The listing builds one solid part. Answer for the finished solid, in the listing's coordinates (mm). Face numbers are marked on the shaded views. A direction names the side the tool comes from. Round coordinates to 2 decimals unless told otherwise and drop trailing zeros. Write each loop counter-clockwise with the first axis right and the second up, starting at its lowest first coordinate (ties: lowest second). Pieces come first, ordered by that corner, then holes.
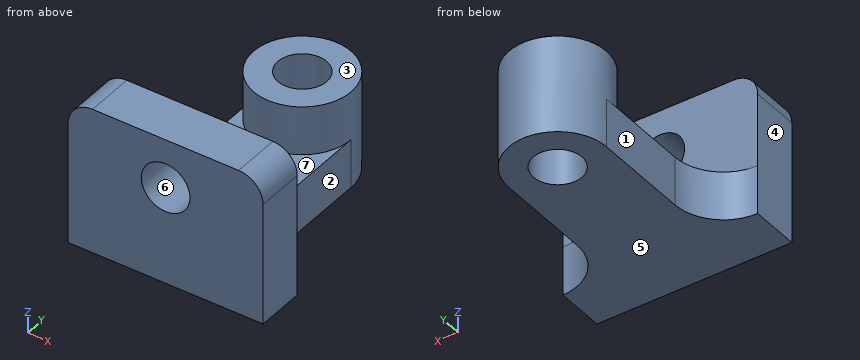
Autodesk Inventor part; units mm, degrees
ref_plane "YZ Plane" through (0, 0, 0) normal (1, 0, 0) x (0, 1, 0)
ref_plane "XZ Plane" through (0, 0, 0) normal (0, 1, 0) x (-1, 0, 0)
ref_plane "XY Plane" through (0, 0, 0) normal (0, 0, 1) x (1, 0, 0)
sketch "Sketch1" plane through (0, 0, 0) normal (0, 1, 0) x (-1, 0, 0)
  line L0 (28.0719, 23.0631) -> (-22.7281, 23.0631)
  line L1 (-22.7281, 23.0631) -> (-22.7281, -15.0369)
  line L2 (-22.7281, -15.0369) -> (28.0719, -15.0369)
  line L3 (28.0719, -15.0369) -> (28.0719, 23.0631)
  point P0 (0, 0)
  dimension "d0" = 50.8
  dimension "d1" = 38.1
extrude "Extrusion1" add sketch "Sketch1" along normal blind 12.7
sketch "Sketch2" plane through (0, 12.7, 0) normal (0, 1, 0) x (1, 0, 0)
  line L0 (22.7281, -23.0631) -> (22.7281, 15.0369)
  line L1 (22.7281, 15.0369) -> (10.0281, 15.0369)
  line L2 (10.0281, 15.0369) -> (10.0281, 2.3369)
  line L3 (10.0281, 2.3369) -> (22.7281, 2.3369)
  line L4 (22.7281, 2.3369) -> (22.7281, 15.0369)
  line L5 (22.7281, 15.0369) -> (-28.0719, 15.0369)
  line L6 (-28.0719, 15.0369) -> (-15.3719, 15.0369)
  line L7 (-15.3719, 15.0369) -> (-15.3719, 2.3369)
  line L8 (-15.3719, 2.3369) -> (-28.0719, 2.3369)
  line L9 (-28.0719, 2.3369) -> (-28.0719, 15.0369)
  line L10 (-15.3719, 15.0369) -> (10.0281, 15.0369)
  line L11 (10.0281, 15.0369) -> (10.0281, 2.3369)
  line L12 (10.0281, 2.3369) -> (-15.3719, 2.3369)
  line L13 (-15.3719, 2.3369) -> (-15.3719, 15.0369)
  point P0 (0, 0)
  dimension "d4" = 12.7
  dimension "d5" = 12.7
  dimension "d6" = 12.7
  dimension "d7" = 12.7
extrude "Extrusion2" add sketch "Sketch2" along normal blind 38.1 contours L12 L7 L5 L2
fillet "Fillet1" radius 12.7 1 edges at (10.0281, 12.7, -8.6869)
fillet "Fillet2" radius 12.7 1 edges at (-15.3719, 12.7, -8.6869)
sketch "Sketch3" plane through (22.7281, 0, -15.0369) normal (0, 0, -1) x (-1, 0, 0)
  line L0 (12.7, 25.4) -> (12.7, 50.8)
  line L1 (12.7, 50.8) -> (25.4, 50.8)
  line L2 (12.7, 50.8) -> (38.1, 50.8)
  circle A0 centre (25.4, 50.8) radius 12.7
  point P0 (22.7281, 0)
  dimension "d12" = 12.7
  dimension "d13" = 25.4
extrude "Extrusion3" add sketch "Sketch3" against normal blind 25.4
sketch "Sketch4" plane through (-2.6719, 50.8, 10.3631) normal (0, 0, 1) x (1, 0, 0)
  circle A0 centre (0, 0) radius 6.35
  point P0 (2.6719, -50.8)
  dimension "d16" = 12.7
extrude "Extrusion4" cut sketch "Sketch4" against normal blind 25.4
fillet "Fillet3" radius 6.35 1 edges at (22.7281, 6.35, 23.0631)
fillet "Fillet4" radius 6.35 1 edges at (-28.0719, 6.35, 23.0631)
sketch "Sketch6" plane through (0, 12.7, 0) normal (0, 1, 0) x (1, 0, 0)
  line L0 (-21.7219, -23.0631) -> (16.3781, -23.0631)
  line L1 (-2.6719, -23.0631) -> (-2.6719, -10.3631)
  circle A0 centre (-2.6719, -10.3631) radius 6.35
  point P0 (0, 0)
  dimension "d22" = 12.7
  dimension "d23" = 12.7
extrude "Extrusion5" cut sketch "Sketch6" against normal blind 25.4
1. Straight lines are drawn through the part: line 1 along X through (y, z) = (5, 10); line 2 along Y through (x, z) = (1.5, 4.5); line 3 along Y through (x, z) = (-20, 6.5). For each, find the intervals that lie inside material, in ascending order.
Geometry says:
line 1: x = -28.07 to -9.01, 3.67 to 22.73
line 2: y = 0 to 12.7, 38.8 to 46.01, 55.59 to 62.8
line 3: y = 0 to 12.7
2. For a pull along Z with two mould halves and no side action, classify the marked faces 4, 5, 6 and 7 as released by +Z, released by -Z, zero draft, split by the parting line, or undercut.
Geometry says:
face 4: zero draft
face 5: released by -Z
face 6: undercut
face 7: released by +Z
3. Given pin 1 (6.5 mm diameter, centred on y = 40, z = -6.5, fed in from -X); pin 2 (11.5 mm diameter, centred on x = -2.67, z = 10.36, fed in from -Y); pin 3 (5 mm diameter, centred on x = 4, z = 9, fed in from -Y); pin 4 (2 mm diameter, centred on x = 10, z = 18.5, fed in from +Y), each flat-ended and moving along its own axis, determine where each tip first touches the part or whether it passes through.
Geometry says:
pin 1: stops at x = -15.37
pin 2: stops at y = 38.1
pin 3: stops at y = 0
pin 4: stops at y = 12.7
4. Section D-D on y = 37 is taken. Determine the outline of the cut face in (x, z).
Geometry says:
outline: (-15.37, -15.04) - (10.03, -15.04) - (10.03, -2.34) - (-15.37, -2.34) - close
5. Section B-B on x = -3 is taken. Determine the outline of the cut face in (y, z).
Geometry says:
outline: (0, -15.04) - (44.46, -15.04) - (44.46, 10.36) - (38.1, 10.36) - (38.1, -2.34) - (12.7, -2.34) - (12.7, 4.02) - (0, 4.02) - close; (0, 16.7) - (12.7, 16.7) - (12.7, 23.06) - (0, 23.06) - close; (57.14, -15.04) - (63.5, -15.04) - (63.5, 10.36) - (57.14, 10.36) - close
6. A tool of negligible diameter and unlimited length cuts with its end or side. For the marked faces 1, 2 and 3, from which of +Z, -Z, +X, -X, +Y, -Y can it reach the whole face along a straight path? Write none if from no direction.
Geometry says:
face 1: +Z, -Z, -X, +Y
face 2: +Z, -Z, +X, +Y
face 3: +Z, +X, -X, +Y
7. Section C-C on z = 15 is taken. Determine the outline of the cut face in (x, y).
Geometry says:
outline: (-28.07, 0) - (-7.01, 0) - (-7.01, 12.7) - (-28.07, 12.7) - close; (1.67, 0) - (22.73, 0) - (22.73, 12.7) - (1.67, 12.7) - close
